CAD build for the part. Positions are in the model's coordinates, mm. A direction names the side the tool comes from. Coordinates: 2 decimals unless noted, no trailing zeros. Order: outer loops, then holes, each group sorted by start corner. A loop starts at its lowest first (then second) coordinate and runs counter-clockwise, first axis right, second up. Notation, with made-up numbers: (37, -33) - (72, -33) arc R10 cw to (72, -22) - close; hole circle Ø2 at (6.5, 85). An arc over 180 degrees is marked (long way). Return JSON: item names as keys, results as strings.
from build123d import *

# Parameters (mm, degrees)
ESQUISSE1_R                  = 0.7499999999999986
ESQUISSE1_R_2                = 1.050000000000001
BOSS_EXTRU_1_DEPTH           = 5.588
BOSS_EXTRU_2_DEPTH           = 11.43
ENL_V_MAT_EXTRU_1_DEPTH      = 3.5
ENL_V_MAT_EXTRU_1_DEPTH_BACK = 3.5
CONG_1_R                     = 7
CONG_2_R                     = 2
ESQUISSE5_R                  = 1.0500000000000025
ENL_V_MAT_EXTRU_2_DEPTH      = 59.98362409134528


with BuildPart() as part:
    # Esquisse1 → Boss.-Extru.1 (new body)
    with BuildSketch(Plane(origin=(0, 0, 0), x_dir=(0, 0, -1), z_dir=(1, 0, 0))):
        with BuildLine():
            ThreePointArc((-34.6, 0), (-29.084530777641156, 18.741666666666667), (-14.296527777777778, 31.508241675777914))
            ThreePointArc((-14.296527777777778, 31.508241675777914), (-12.55545845283557, 36.141672111831234), (-17.18888888888889, 37.88274143677345))
            ThreePointArc((-17.18888888888889, 37.88274143677345), (-34.968684403175494, 22.53333333333333), (-41.6, 0))
            ThreePointArc((-41.6, 0), (-38.1, -3.5), (-34.6, 0))
        make_face()
        with Locations((-38.1, 0)):
            Circle(ESQUISSE1_R, mode=Mode.SUBTRACT)
        with Locations((-15.742708333333335, 34.69549155627568)):
            Circle(ESQUISSE1_R_2, mode=Mode.SUBTRACT)
    extrude(amount=BOSS_EXTRU_1_DEPTH)

    # Esquisse2 → Boss.-Extru.2 (add)
    with BuildSketch(Plane(origin=(5.588, 0, 0), x_dir=(0, 0, -1), z_dir=(1, 0, 0))):
        with BuildLine():
            Line((-21.515108455003254, 27.09723432694649), (-25.765862615540357, 32.66007231585839))
            ThreePointArc((-25.765862615540357, 32.66007231585839), (-21.63554338093815, 35.53115903839253), (-17.188888888888894, 37.88274143677345))
            ThreePointArc((-17.188888888888894, 37.88274143677345), (-12.555458452835564, 36.141672111831234), (-14.296527777777776, 31.508241675777906))
            ThreePointArc((-14.296527777777776, 31.508241675777906), (-18.04113546523944, 29.52418383503393), (-21.515108455003254, 27.09723432694649))
        make_face()
    extrude(amount=BOSS_EXTRU_2_DEPTH)

    # Esquisse4 → Enlèv. mat.-Extru.1 (cut, two sides: drawn at the far end of the back side and taken through both)
    with BuildSketch(Plane(origin=(8.762999999999998, 0, 0), x_dir=(0, 0, -1), z_dir=(1, 0, 0)).offset(-ENL_V_MAT_EXTRU_1_DEPTH_BACK)):
        with BuildLine():
            Line((-22.940194161396708, 34.703133746643395), (-19.080065336161688, 28.86366412581397))
            ThreePointArc((-19.080065336161688, 28.86366412581397), (-16.740600036372985, 30.28055994234895), (-14.296527777777776, 31.508241675777906))
            ThreePointArc((-14.296527777777776, 31.508241675777906), (-12.555458452835564, 36.141672111831234), (-17.188888888888894, 37.88274143677345))
            ThreePointArc((-17.188888888888894, 37.88274143677345), (-20.127426633327065, 36.40668478617679), (-22.940194161396708, 34.703133746643395))
        make_face()
    extrude(amount=ENL_V_MAT_EXTRU_1_DEPTH + ENL_V_MAT_EXTRU_1_DEPTH_BACK, mode=Mode.SUBTRACT)

    # Congé1
    cong_1_edges = [part.edges().sort_by_distance(p)[0] for p in [
        (5.588, 29.878653321402442, 23.640485535271807),
    ]]
    fillet(cong_1_edges, radius=CONG_1_R)

    # Congé2
    cong_2_edges = [part.edges().sort_by_distance(p)[0] for p in [
        (17.018, 29.878653321402442, 23.640485535271807),
    ]]
    fillet(cong_2_edges, radius=CONG_2_R)

    # Esquisse5 → Enlèv. mat.-Extru.2 (cut, through all)
    with BuildSketch(Plane.ZY):
        with Locations(Location((15.742708333333335, 34.69549155627568, 0), (0, 0, 180))):
            Circle(ESQUISSE5_R)
    extrude(amount=-ENL_V_MAT_EXTRU_2_DEPTH, mode=Mode.SUBTRACT)


solid = part.part
Item 1: Band-saw the part on A-A, the plane z = 38.1. List the corners of the cut face in (x, y).
Findings below:
{"outline": "(0, -3.5) - (5.59, -3.5) - (5.59, -0.75) - (0, -0.75) - close; (0, 0.75) - (5.59, 0.75) - (5.59, 16.7) - (0, 16.7) - close"}
Item 2: Drop flat-ended pins along their axis: P1, Ø1.3, axis at y = 0, z = 38.1, coming from the -X side; P2, Ø3, axis at x = 7, z = 20.5, coming from the -Y side; P3, Ø16.5, axis at y = 7, z = 32, coming from the +X side; P4, Ø10, axis at x = 5.5, z = 20, coming from the -Y side. Give the stop position or say it passes through.
Findings below:
{"P1": "passes through", "P2": "stops at y = 26.71", "P3": "stops at x = 5.59", "P4": "stops at y = 23.92"}
Item 3: Which spindle directions (+Z, -Z, +X, -X, +Y, -Y) get a long thin tool onto all of the face, cutting with end or side? Do faces 1 (the flat face through (0, 21, 29)), 2 (the flat face through (5.263, 34, 18)), 3 (the flat face through (13.79, 29.84, 23.61)). Say none if no direction does.
Findings below:
{"face 1": "+Z, -Z, -X, +Y, -Y", "face 2": "-Z, +Y", "face 3": "+Z, +X, -Y"}
Item 4: Wall check: L1, parallel to X at y = 34.5, z = 17.5; L2, parallel to X at y = 22.5, z = 30.25; L3, parallel to Y at x = 3.65, z = 38.1. Give the ranges that are in metal, low to high. Write a range as [from, to].
Findings below:
{"L1": "x = [0, 5.26], [12.26, 17.02]", "L2": "x = [0, 5.59]", "L3": "y = [-3.5, -0.75], [0.75, 16.7]"}
Item 5: Mould opens along Y. For faces 4 (the flat face through (12.263, 34, 18)), 5 (the cylindrical face through (14.61, 33.81, 15.18)), 6 (the cylindrical face through (2.8, -3.5, 38.2)) say: released by +Y, released by -Y, zero draft, split by the parting line, or undercut.
Findings below:
{"face 4": "zero draft", "face 5": "undercut", "face 6": "released by -Y"}
Item 6: Band-saw the part on C-C, the plane x = 10.25. List the corners of the cut face in (y, z).
Findings below:
{"outline": "(26.85, 21.83) arc R34.6 cw to (28.86, 19.08) - (34.7, 22.94) arc R41.6 ccw to (32.41, 26.08) - close"}
